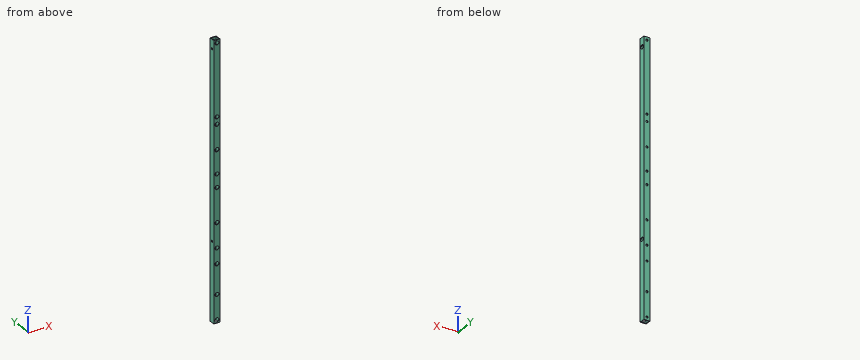
from build123d import *

# Parameters (mm, degrees)
SKETCH_1_W                  = 15
SKETCH_1_H                  = 15
SKETCH_1_W_2                = 12
SKETCH_1_H_2                = 12
EXTRUDE_1_DEPTH             = 670
SKETCH_4_R                  = 2.7
CUT_EXTRUDE_3_DEPTH         = 20
SKETCH_3_R                  = 2.7
CUT_EXTRUDE_4_DEPTH         = 30
SKETCH_5_R                  = 2.7
CUT_EXTRUDE_5_DEPTH         = 40
SKETCH_6_R                  = 5
CUT_EXTRUDE_6_DEPTH         = 10
SKETCH_7_R                  = 5
CUT_EXTRUDE_7_DEPTH         = 10
HOLE_WIZARD_5_4_5_4_1_D     = 5.4
HOLE_WIZARD_10_0_10_1_D     = 10
HOLE_WIZARD_10_0_10_1_DEPTH = 1.5
HOLE_WIZARD_10_0_10_1_TIP   = 3.004303095


with BuildPart() as part:
    # ｽｹｯﾁ1 → ﾎﾞｽ - 押し出し1 (new body)
    with BuildSketch(Plane.XY):
        Rectangle(SKETCH_1_W, SKETCH_1_H)
        Rectangle(SKETCH_1_W_2, SKETCH_1_H_2, mode=Mode.SUBTRACT)
    extrude(amount=EXTRUDE_1_DEPTH)

    # ｽｹｯﾁ4 → ｶｯﾄ - 押し出し3 (cut)
    with BuildSketch(Plane(origin=(7.5, 0, 0), x_dir=(0, 0, -1), z_dir=(1, 0, 0))):
        with Locations((-647.5, 0)):
            Circle(SKETCH_4_R)
        with Locations((-192.5, 0)):
            Circle(SKETCH_4_R)
    extrude(amount=-CUT_EXTRUDE_3_DEPTH, mode=Mode.SUBTRACT)

    # ｽｹｯﾁ3 → ｶｯﾄ - 押し出し4 (cut)
    with BuildSketch(Plane(origin=(0, 7.5, 0), x_dir=(1, 0, 0), z_dir=(0, 1, 0))):
        with Locations((0, -177.5)):
            Circle(SKETCH_3_R)
        with Locations((0, -487.5)):
            Circle(SKETCH_3_R)
        with Locations((0, -352.5)):
            Circle(SKETCH_3_R)
        with Locations((0, -662.5)):
            Circle(SKETCH_3_R)
        with Locations((0, -140)):
            Circle(SKETCH_3_R)
    extrude(amount=-CUT_EXTRUDE_4_DEPTH, mode=Mode.SUBTRACT)

    # ｽｹｯﾁ5 → ｶｯﾄ - 押し出し5 (cut)
    with BuildSketch(Plane(origin=(0, 7.5, 0), x_dir=(1, 0, 0), z_dir=(0, 1, 0))):
        with Locations((0, -7.5)):
            Circle(SKETCH_5_R)
        with Locations((0, -67.5)):
            Circle(SKETCH_5_R)
        with Locations((0, -410)):
            Circle(SKETCH_5_R)
        with Locations((0, -470)):
            Circle(SKETCH_5_R)
    extrude(amount=-CUT_EXTRUDE_5_DEPTH, mode=Mode.SUBTRACT)

    # ｽｹｯﾁ6 → ｶｯﾄ - 押し出し6 (cut)
    with BuildSketch(Plane(origin=(0, -7.5, 0), x_dir=(-1, 0, 0), z_dir=(0, -1, 0))):
        with Locations((0, -662.5)):
            Circle(SKETCH_6_R)
        with Locations((0, -177.5)):
            Circle(SKETCH_6_R)
        with Locations((0, -352.5)):
            Circle(SKETCH_6_R)
        with Locations((0, -487.5)):
            Circle(SKETCH_6_R)
        with Locations((0, -470)):
            Circle(SKETCH_6_R)
        with Locations((0, -410)):
            Circle(SKETCH_6_R)
        with Locations((0, -67.5)):
            Circle(SKETCH_6_R)
        with Locations((0, -7.5)):
            Circle(SKETCH_6_R)
        with Locations((0, -140)):
            Circle(SKETCH_6_R)
    extrude(amount=-CUT_EXTRUDE_6_DEPTH, mode=Mode.SUBTRACT)

    # ｽｹｯﾁ7 → ｶｯﾄ - 押し出し7 (cut)
    with BuildSketch(Plane(origin=(7.5, 0, 0), x_dir=(0, 0, -1), z_dir=(1, 0, 0))):
        with Locations((-647.5, 0)):
            Circle(SKETCH_7_R)
        with Locations((-192.5, 0)):
            Circle(SKETCH_7_R)
    extrude(amount=-CUT_EXTRUDE_7_DEPTH, mode=Mode.SUBTRACT)

    # Ø5.4 (5.4) 直径の穴1 (through all)
    with Locations(Plane(origin=(0, 7.5, 0), x_dir=(1, 0, 0), z_dir=(0, 1, 0))):
        with Locations((0, -237.5), (0, -320.5)):
            Hole(HOLE_WIZARD_5_4_5_4_1_D / 2)

    # Ø10.0 (10) 直径の穴1
    with Locations(Plane(origin=(0, -7.5, 0), x_dir=(-1, 0, 0), z_dir=(0, -1, 0))):
        with Locations((0, -237.5), (0, -320.5)):
            Hole(HOLE_WIZARD_10_0_10_1_D / 2, depth=HOLE_WIZARD_10_0_10_1_DEPTH)
            with Locations((0, 0, -(HOLE_WIZARD_10_0_10_1_DEPTH + HOLE_WIZARD_10_0_10_1_TIP / 2))):  # 118° drill point
                Cone(0, HOLE_WIZARD_10_0_10_1_D / 2, HOLE_WIZARD_10_0_10_1_TIP, mode=Mode.SUBTRACT)


solid = part.part
Can you work these out from the model? Positions are in its coordinate system, mm. Coordinates: 2 decimals unless noted, no trailing zeros. Loops run counter-clockwise (first coordinate to the right, second up) from the corner with the lowest first, then second, coordinate; pieces in that order, holes last. Notation, with made-up numbers: (73, 23.5) - (106, 23.5) arc R21 ccw to (106, 53.5) - close; hole circle Ø6 at (46.5, 86). An arc over 180 degrees is marked (long way). Put each result on its own line as item: value. Start each with the question number.
Item 1: For pin 1 (6 mm diameter, centred on x = 0, z = 7.5, fed in from -Y); pin 2 (3 mm diameter, centred on x = 0, z = 320.5, fed in from +Y), each with a flat end and sliding along its axis, tell me the tip position at first contact or that it passes through.
Item 2: If I drill on line 1 along X through (y, z) = (6.7, 487.5); line 2 along X through (y, z) = (2, 482.5), over which ranges is the centre line in solid material (lowest first)?
Item 3: Suppose I cut it at A-A (z = 102). Please give me the cut outline in (x, y).
Item 4: Suppose I cut it at B-B (x = 0). State how many separate pieces and enclosed holes the cut face has, and give its area (3 significant figures).
Here are the results:
1. pin 1: y = 6
1. pin 2: through
2. line 1: -7.5 to -2.7, 2.7 to 7.5
2. line 2: -7.5 to -6, 6 to 7.5
3. outline: (-7.5, -7.5) - (7.5, -7.5) - (7.5, 7.5) - (-7.5, 7.5) - close; hole (-6, -6) - (6, -6) - (6, 6) - (-6, 6) - close
4. separate pieces: 24
4. enclosed holes: 0
4. area: 1,760 mm²
